Read the model definition and answer for the solid it produces. Units are mm, in the model's axes. Give positions to 0.01 mm unless a question says otherwise; leave off trailing zeros. Loops run counter-clockwise (first coordinate to the right, second up) from the corner with the lowest first, then second, coordinate; pieces in that order, holes last. Notation, with made-up numbers: M 17.25,-20.75 L 51.25,-20.75 A24 cw 51.25,1.25 Z; hole C -12,75 d6. An arc over 180 degrees is marked long. Return JSON: item names as keys, results as strings. Group by question number.
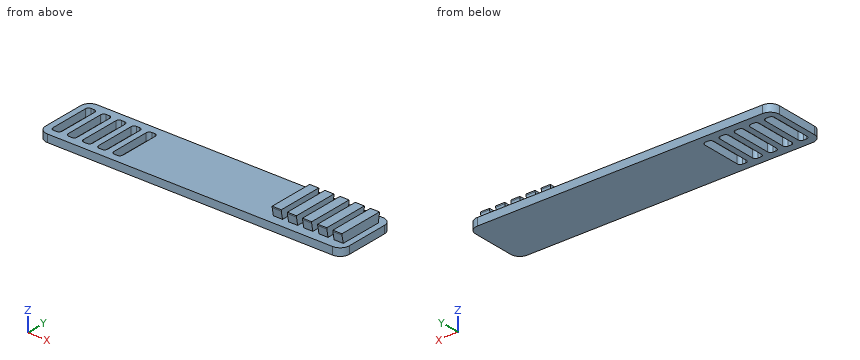
```python
from build123d import *

# Parameters (mm, degrees)
F0_W     = 100
F0_H     = 20
F0_W_2   = 3
F0_H_2   = 15
F1_DEPTH = 2.5
F2_W     = 3
F2_H     = 15
F3_DEPTH = 3
F5_DEPTH = 98.001
F6_R     = 3


# Not quite as in the source:
# - a feature names something its author has since deleted; it is built from what else it names


with BuildPart() as f1:
    # F0 (on Top) → F1 (new body)
    with BuildSketch(Plane.XY):
        Rectangle(F0_W, F0_H)
        with BuildLine():
            ThreePointArc((-45, -6.5), (-45.2928932188, -7.2071067812), (-46, -7.5))
            Line((-46, -7.5), (-47, -7.5))
            ThreePointArc((-47, -7.5), (-47.7071067812, -7.2071067812), (-48, -6.5))
            Line((-48, -6.5), (-48, 6.5))
            ThreePointArc((-48, 6.5), (-47.7071067812, 7.2071067812), (-47, 7.5))
            Line((-47, 7.5), (-46, 7.5))
            ThreePointArc((-46, 7.5), (-45.2928932188, 7.2071067812), (-45, 6.5))
            Line((-45, 6.5), (-45, -6.5))
        make_face(mode=Mode.SUBTRACT)
        with BuildLine():
            Line((-42, 7.5), (-41, 7.5))
            ThreePointArc((-41, 7.5), (-40.2928932188, 7.2071067812), (-40, 6.5))
            Line((-40, 6.5), (-40, -6.5))
            ThreePointArc((-40, -6.5), (-40.2928932188, -7.2071067812), (-41, -7.5))
            Line((-41, -7.5), (-42, -7.5))
            ThreePointArc((-42, -7.5), (-42.7071067812, -7.2071067812), (-43, -6.5))
            Line((-43, -6.5), (-43, 6.5))
            ThreePointArc((-43, 6.5), (-42.7071067812, 7.2071067812), (-42, 7.5))
        make_face(mode=Mode.SUBTRACT)
        with BuildLine():
            Line((-37, 7.5), (-36, 7.5))
            ThreePointArc((-36, 7.5), (-35.2928932188, 7.2071067812), (-35, 6.5))
            Line((-35, 6.5), (-35, -6.5))
            ThreePointArc((-35, -6.5), (-35.2928932188, -7.2071067812), (-36, -7.5))
            Line((-36, -7.5), (-37, -7.5))
            ThreePointArc((-37, -7.5), (-37.7071067812, -7.2071067812), (-38, -6.5))
            Line((-38, -6.5), (-38, 6.5))
            ThreePointArc((-38, 6.5), (-37.7071067812, 7.2071067812), (-37, 7.5))
        make_face(mode=Mode.SUBTRACT)
        with BuildLine():
            Line((-32, 7.5), (-31, 7.5))
            ThreePointArc((-31, 7.5), (-30.2928932188, 7.2071067812), (-30, 6.5))
            Line((-30, 6.5), (-30, -6.5))
            ThreePointArc((-30, -6.5), (-30.2928932188, -7.2071067812), (-31, -7.5))
            Line((-31, -7.5), (-32, -7.5))
            ThreePointArc((-32, -7.5), (-32.7071067812, -7.2071067812), (-33, -6.5))
            Line((-33, -6.5), (-33, 6.5))
            ThreePointArc((-33, 6.5), (-32.7071067812, 7.2071067812), (-32, 7.5))
        make_face(mode=Mode.SUBTRACT)
        with BuildLine():
            Line((-27, 7.5), (-26, 7.5))
            ThreePointArc((-26, 7.5), (-25.2928932188, 7.2071067812), (-25, 6.5))
            Line((-25, 6.5), (-25, -6.5))
            ThreePointArc((-25, -6.5), (-25.2928932188, -7.2071067812), (-26, -7.5))
            Line((-26, -7.5), (-27, -7.5))
            ThreePointArc((-27, -7.5), (-27.7071067812, -7.2071067812), (-28, -6.5))
            Line((-28, -6.5), (-28, 6.5))
            ThreePointArc((-28, 6.5), (-27.7071067812, 7.2071067812), (-27, 7.5))
        make_face(mode=Mode.SUBTRACT)
        with Locations((26.5, 0)):
            Rectangle(F0_W_2, F0_H_2, mode=Mode.SUBTRACT)
        with Locations((31.5, 0)):
            Rectangle(F0_W_2, F0_H_2, mode=Mode.SUBTRACT)
        with Locations((36.5, 0)):
            Rectangle(F0_W_2, F0_H_2, mode=Mode.SUBTRACT)
        with Locations((41.5, 0)):
            Rectangle(F0_W_2, F0_H_2, mode=Mode.SUBTRACT)
        with Locations((46.5, 0)):
            Rectangle(F0_W_2, F0_H_2, mode=Mode.SUBTRACT)
        with Locations((26.5, 0)):
            Rectangle(F0_W_2, F0_H_2)
        with Locations((31.5, 0)):
            Rectangle(F0_W_2, F0_H_2)
        with Locations((36.5, 0)):
            Rectangle(F0_W_2, F0_H_2)
        with Locations((41.5, 0)):
            Rectangle(F0_W_2, F0_H_2)
        with Locations((46.5, 0)):
            Rectangle(F0_W_2, F0_H_2)
    extrude(amount=F1_DEPTH)

    # F2 (on face) → F3 (join)
    with BuildSketch(Plane.XY.offset(2.5)):
        with Locations((26.5, 0)):
            Rectangle(F2_W, F2_H)
        with Locations((31.5, 0)):
            Rectangle(F2_W, F2_H)
        with Locations((36.5, 0)):
            Rectangle(F2_W, F2_H)
        with Locations((41.5, 0)):
            Rectangle(F2_W, F2_H)
        with Locations((46.5, 0)):
            Rectangle(F2_W, F2_H)
    extrude(amount=F3_DEPTH)

    # F4 (on face) → F5 (cut, through all)
    with BuildSketch(Plane.YZ.offset(48)):
        Polygon((-7.5, 5.1), (-7.5, 2.5), (-7, 2.5), align=None)
        Polygon((7.5, 5.1), (7, 2.5), (7.5, 2.5), align=None)
    extrude(amount=-F5_DEPTH, mode=Mode.SUBTRACT)

    # F6
    f6_edges = [f1.edges().sort_by_distance(p)[0] for p in [
        (-50, -10, 1.25),
        (50, -10, 1.25),
        (-50, 10, 1.25),
        (50, 10, 1.25),
    ]]
    fillet(f6_edges, radius=F6_R)


solid = f1.part
```
1. Find section B-B (z = 3.85). Write down the section's boundary in (x, y), and give its area (3 significant figures).
2. Flat-ended cylindrical pins translate along their axes: P1, Ø2, axis at y = 7, z = 4.5, coming from the +X side; P2, Ø5, axis at x = -38, y = -0.5, coming from the +Z side; P3, Ø0.9, axis at y = 0, z = 3.5, coming from the -X side. Find the tip coordinate at first contact, or state that the pin passes through.
3. Find section A-A (y = 0.75). State how many separate pieces and enclosed holes the cut face has, and give its area (4 significant figures).
4. Straight lines are drawn through the part: line 1 along X through (y, z) = (0, 4.55); line 2 along X through (y, z) = (2, 0.8); line 3 along Y through (x, z) = (-32, 0.85). For each, find the intervals that lie inside material, in ascending order.
5. Find section C-C (x = 26.5). Write down the section's boundary in (y, z).
6. Find section D-D (x = 8.5). Write down the section's boundary in (y, z).
Result:
{
 "1": {"outline": "M 25,-7.26 L 28,-7.26 L 28,7.26 L 25,7.26 Z; M 30,-7.26 L 33,-7.26 L 33,7.26 L 30,7.26 Z; M 35,-7.26 L 38,-7.26 L 38,7.26 L 35,7.26 Z; M 40,-7.26 L 43,-7.26 L 43,7.26 L 40,7.26 Z; M 45,-7.26 L 48,-7.26 L 48,7.26 L 45,7.26 Z", "area": "218 mm2"},
 "2": {"P1": "stops at x = 48", "P2": "stops at z = 2.5", "P3": "stops at x = 25"},
 "3": {"separate pieces": "6", "enclosed holes": "0", "area": "257.5 mm2"},
 "4": {"line 1": "x = 25 to 28, 30 to 33, 35 to 38, 40 to 43, 45 to 48", "line 2": "x = -50 to -48, -45 to -43, -40 to -38, -35 to -33, -30 to -28, -25 to 50", "line 3": "y = -10 to -7.5, 7.5 to 10"},
 "5": {"outline": "M -10,0 L 10,0 L 10,2.5 L 7,2.5 L 7.5,5.1 L 7.5,5.5 L -7.5,5.5 L -7.5,5.1 L -7,2.5 L -10,2.5 Z"},
 "6": {"outline": "M -10,0 L 10,0 L 10,2.5 L -10,2.5 Z"}
}
